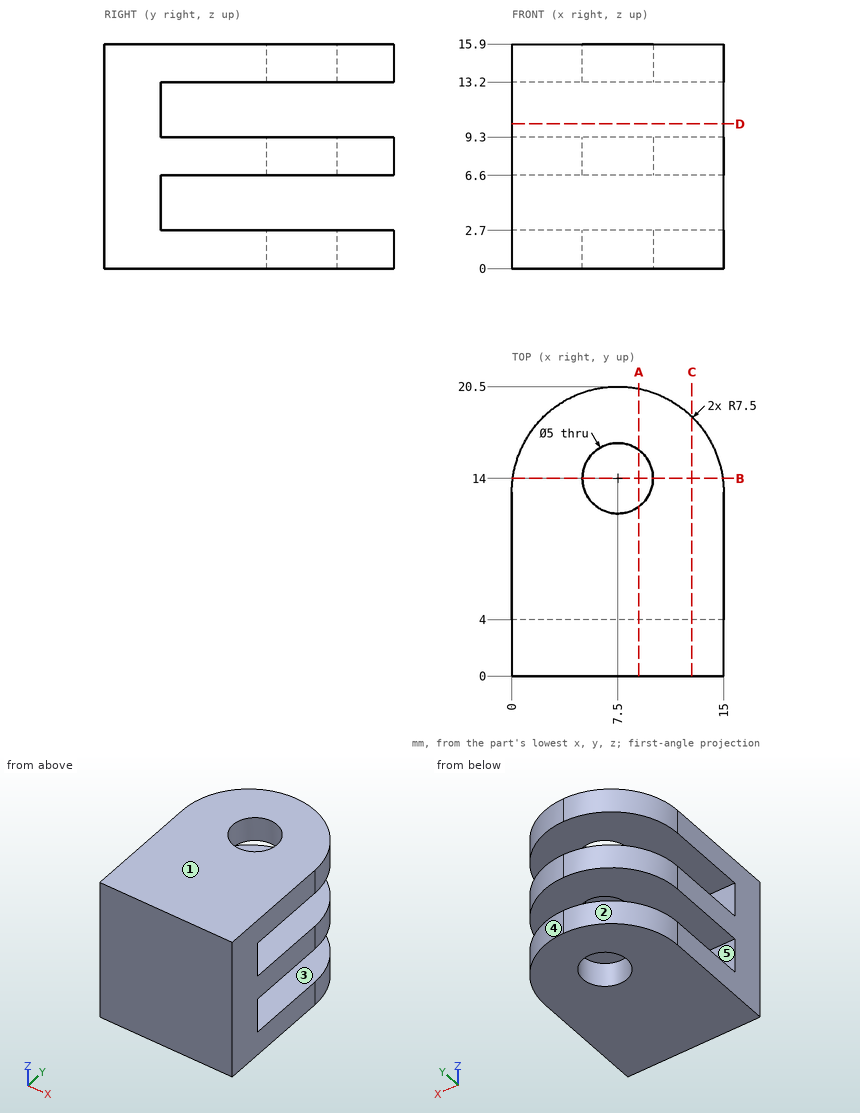
Geometry check sheet. Reference: drawing and pictorial views, mm from the part's lowest x, y, z. A direction names the side the tool comes from. Coordinates: 2 decimals unless noted, no trailing zeros. Order: outer loops, then holes, each group sorted by start corner. A loop starts at its lowest first (then second) coordinate and runs counter-clockwise, first axis right, second up. Notation, with made-up numbers: (76.25, -29.75) -> (90.25, -29.75) arc R33 cw to (90.25, 3.25) -> close; hole circle Ø9 at (2, -28.5). An arc over 180 degrees is marked (long way). Use CSV: the item, a comma, the result in double quotes. Start each with the question number.
Q1. Draft check along Z on the marked faces 1, 2 and 3. Enter one of: +Z half, -Z half, draft (parallel to the pull), parting line (faces both ways), or undercut.
Q2. Depth check by flat-ended pin: P1, Ø1.2, axis at x = 10, z = 4, coming from the +Y side; P2, Ø4, axis at x = 7.5, y = 14, coming from the -Z side (1 decimal). Enter the tip coordinate at first touch or a pass-through.
Q3. Section check A-A, the plane x = 9. Record the cut outline in (y, z).
Q4. Section check B-B, the plane y = 14. Record the cut outline in (x, z).
Q5. Section check C-C, the plane x = 12.75. Record the cut outline in (y, z), and give its area (3 significant figures).
Q6. Section check D-D, the plane z = 10.25. Record the cut outline in (x, y), and give its area (3 significant figures).
Q7. Tool access check on the marked faces 4 and 5. Record the directions out of +Z, -Z, +X, -X, +Y, -Y that give a thin tool (end or side, any length) a straight path to the whole face; none if there is none.
Q8. Thickness scan on line 1 along Z through (x, y) = (7.75, 18.5); line 2 along Y through (x, z) = (7.5, 13.9); line 3 along Y through (x, z) = (7.5, 6.25). Record the ranges inside material, lowest first.
Returned:
1,face 1,"+Z half"
1,face 2,"draft"
1,face 3,"undercut"
2,P1,"stops at y = 4"
2,P2,"passes through"
3,outline,"(0, 0) -> (12, 0) -> (12, 2.7) -> (4, 2.7) -> (4, 6.6) -> (12, 6.6) -> (12, 9.3) -> (4, 9.3) -> (4, 13.2) -> (12, 13.2) -> (12, 15.9) -> (0, 15.9) -> close; (16, 0) -> (20.35, 0) -> (20.35, 2.7) -> (16, 2.7) -> close; (16, 6.6) -> (20.35, 6.6) -> (20.35, 9.3) -> (16, 9.3) -> close; (16, 13.2) -> (20.35, 13.2) -> (20.35, 15.9) -> (16, 15.9) -> close"
4,outline,"(0.07, 0) -> (5, 0) -> (5, 2.7) -> (0.07, 2.7) -> close; (0.07, 6.6) -> (5, 6.6) -> (5, 9.3) -> (0.07, 9.3) -> close; (0.07, 13.2) -> (5, 13.2) -> (5, 15.9) -> (0.07, 15.9) -> close; (10, 0) -> (14.93, 0) -> (14.93, 2.7) -> (10, 2.7) -> close; (10, 6.6) -> (14.93, 6.6) -> (14.93, 9.3) -> (10, 9.3) -> close; (10, 13.2) -> (14.93, 13.2) -> (14.93, 15.9) -> (10, 15.9) -> close"
5,outline,"(0, 0) -> (18.36, 0) -> (18.36, 2.7) -> (4, 2.7) -> (4, 6.6) -> (18.36, 6.6) -> (18.36, 9.3) -> (4, 9.3) -> (4, 13.2) -> (18.36, 13.2) -> (18.36, 15.9) -> (0, 15.9) -> close"
5,area,"180 mm^2"
6,outline,"(0, 0) -> (15, 0) -> (15, 4) -> (0, 4) -> close"
6,area,"60.0 mm^2"
7,face 4,"+Z, -Z, +X, +Y"
7,face 5,"+X, -X, +Y"
8,line 1,"z = 0 to 2.7, 6.6 to 9.3, 13.2 to 15.9"
8,line 2,"y = 0 to 11.5, 16.5 to 20.5"
8,line 3,"y = 0 to 4"
